Can you work these out from the drawing? Everything is in mm from the part's minimum corner. Give positions to 0.01 mm unless a question says otherwise; leave off trailing zeros. Order: outer loops, then holes, each group sorted by start corner. A loop starts at its lowest first (then second) coordinate and runs counter-clockwise, first axis right, second up. Notation, with made-up numbers: (-15, -18) -> (36, -18) arc R16 ccw to (36, 5) -> close; hole circle Ø4 at (-32.5, -1). An arc over 180 degrees is marked (long way). One line per item, written item: value.
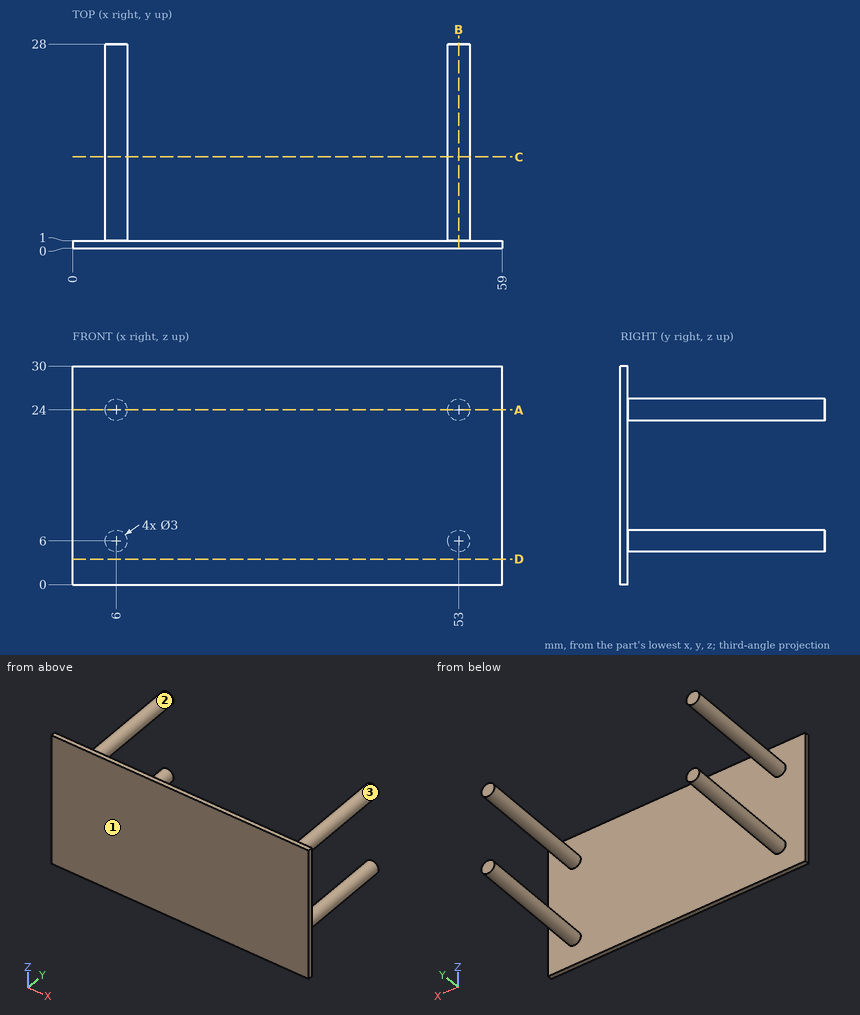
1) Suppose I cut it at A-A, the plane z = 24. Write out the boundary of the cut face in (x, y), then the cut area to 3 significant figures.
Answer below:
outline: (0, 0) -> (59, 0) -> (59, 1) -> (54.5, 1) -> (54.5, 28) -> (51.5, 28) -> (51.5, 1) -> (7.5, 1) -> (7.5, 28) -> (4.5, 28) -> (4.5, 1) -> (0, 1) -> close
area: 221 mm2
2) Suppose I cut it at C-C, the plane y = 12.5. Write out the boundary of the cut face in (x, z).
Answer below:
outline: circle Ø3 at (6, 6); circle Ø3 at (6, 24); circle Ø3 at (53, 6); circle Ø3 at (53, 24)
3) We'd pull the mould along Z, two halves only. Please class the marked faces 1, 2 and 3: +Z half, -Z half, draft (parallel to the pull), parting line (faces both ways), or undercut.
Answer below:
face 1: draft
face 2: undercut
face 3: undercut
4) For P1, Ø4, axis at y = 22.5, z = 24, coming from the -X side; P2, Ø6, axis at y = 23.5, z = 26, coming from the +X side, each with a flat end and sliding along its axis, tell me the tip position at first contact or that it passes through.
Answer below:
P1: stops at x = 4.5
P2: stops at x = 54.5
5) Suppose I cut it at B-B, the plane x = 53. Write out the boundary of the cut face in (y, z), then the cut area to 3 significant figures.
Answer below:
outline: (0, 0) -> (1, 0) -> (1, 4.5) -> (28, 4.5) -> (28, 7.5) -> (1, 7.5) -> (1, 22.5) -> (28, 22.5) -> (28, 25.5) -> (1, 25.5) -> (1, 30) -> (0, 30) -> close
area: 192 mm2
6) Suppose I cut it at D-D, the plane z = 3.5. Write out the boundary of the cut face in (x, y).
Answer below:
outline: (0, 0) -> (59, 0) -> (59, 1) -> (0, 1) -> close
7) If I drill on line 1 along Z through (x, y) = (53, 19.75); line 2 along Y through (x, z) = (10.5, 14.5), over which ranges is the centre line in solid material (lowest first)?
Answer below:
line 1: z = 4.5 to 7.5, 22.5 to 25.5
line 2: y = 0 to 1
